from build123d import *

# Parameters (mm, degrees)
F1_DEPTH = 63.5
F2_DEPTH = 25.4
F3_DEPTH = 7.9375
F4_DEPTH = 25.4


with BuildPart() as f1:
    # F0 (on Front) → F1 (new body, symmetric)
    with BuildSketch(Plane.XZ):
        Polygon((-41.275, 9.525), (-41.275, -9.525), (41.275, -9.525), (41.275, 9.525), (22.225, 9.525), align=None)
    extrude(amount=F1_DEPTH, both=True)

    # F0 (on Front) → F2 (join, symmetric)
    with BuildSketch(Plane.XZ):
        with BuildLine():
            Line((22.225, 9.525), (41.275, 9.525))
            Line((41.275, 9.525), (41.275, 33.834597))
            ThreePointArc((41.275, 33.834597), (43.881091, 40.126257), (50.172751, 42.732348))
            Line((50.172751, 42.732348), (63.788638, 42.732348))
            Line((63.788638, 42.732348), (63.788638, 61.565076))
            Line((63.788638, 61.565076), (77.687105, 61.565076))
            Line((77.687105, 61.565076), (77.685953, 61.782348))
            Line((77.685953, 61.782348), (50.172751, 61.782348))
            ThreePointArc((50.172751, 61.782348), (30.410707, 53.596641), (22.225, 33.834597))
            Line((22.225, 33.834597), (22.225, 9.525))
        make_face()
    extrude(amount=F2_DEPTH, both=True)

    # F0 (on Front) → F3 (join, symmetric)
    with BuildSketch(Plane.XZ):
        with BuildLine():
            add(Edge.make_bspline(
                [(-41.275, 9.525), (-36.848798, 45.56419), (7.302681, 62.255602), (50.172751, 61.782348)],
                knots=[0, 0, 0, 0, 105.325787, 105.325787, 105.325787, 105.325787], degree=3))
            Line((-41.275, 9.525), (22.225, 9.525))
            Line((22.225, 9.525), (22.225, 33.834597))
            ThreePointArc((22.225, 33.834597), (30.410707, 53.596641), (50.172751, 61.782348))
        make_face()
    extrude(amount=F3_DEPTH, both=True)

    # F0 (on Front) → F4 (join, symmetric)
    with BuildSketch(Plane.XZ):
        Polygon((114.588638, 61.565076), (77.687105, 61.565076), (77.837355, 33.214565), (114.588638, 33.214565), align=None)
        Polygon((77.837355, 33.214565), (77.687105, 61.565076), (63.788638, 61.565076), (63.788638, 42.732348), (63.788638, 33.214565), align=None)
    extrude(amount=F4_DEPTH, both=True)


solid = f1.part
Design review of the part built by this model. Coordinates are the model's own, in mm. A direction names the side the tool comes from. Coordinates: 2 decimals unless noted, no trailing zeros. Order: outer loops, then holes, each group sorted by start corner. A loop starts at its lowest first (then second) coordinate and runs counter-clockwise, first axis right, second up.
Item 1: The part is to be moulded in two halves that separate along X. For faces 6 (the flat face through (114.589, 0, 47)), 7 (the cylindrical face through (30.629, 16.547, 53.813)), 8 (the flat face through (89, 0, 33.215)), 9 (the flat face through (57, 0, 42.732)), say which applies: pulls with the +X half, pulls with the -X half, needs draft (parallel to the pull), parting line crosses it, or undercut.
Item 2: For faces 1 (the flat face through (63.789, 0, 38)), 2 (the flat face through (96, 0, 61.565)), 3 (the flat face through (-5, -7.938, 30)), 4 (the flat face through (-5, 7.938, 30)), 5 (the flat face through (68, -25.4, 42)), list the 3-axis set-ups (+Z, -Z, +X, -X, +Y, -Y) from which the entire face can be reached by the end or side of a thin tool; tool diameter is ignored.
Item 3: Take a section at B-B, the plane x = 59. Write out the cut boundary in (y, z).
Item 4: For pin 1 Ø12 at (x, y) = (62.5, -17) entering from -Z; pin 2 Ø10 at (x, z) = (70.5, 31.5) entering from +Y; pin 3 Ø6 at (x, z) = (11, 17) entering from +Y, all flat-tipped, find the tip position at first contact; note any pin that passes through.
Item 5: For line 1 (X direction, y = 17.5, z = 33.5) (3 decimals); line 2 (X direction, y = 20, z = 22.5) (3 decimals); line 3 (Y direction, x = 65.5, z = 49.5), list the stretches that pass through material, from the lowest coordinate up.
Item 6: Take a section at A-A, the plane z = 1. Write out the cut boundary in (x, y) (3 decimals), then the cut area to 3 significant figures.
The answers:
1. face 6: pulls with the +X half
1. face 7: pulls with the -X half
1. face 8: needs draft
1. face 9: undercut
2. face 1: -Z, +Y, -Y
2. face 2: +Z, +X, +Y, -Y
2. face 3: +Z, -X, -Y
2. face 4: +Z, -X, +Y
2. face 5: +Z, +X, -X, -Y
3. outline: (-25.4, 42.73) - (25.4, 42.73) - (25.4, 61.78) - (-25.4, 61.78) - close
4. pin 1: stops at z = 33.21
4. pin 2: stops at y = 25.4
4. pin 3: stops at y = 7.94
5. line 1: x = 22.225 to 41.275, 63.789 to 114.589
5. line 2: x = 22.225 to 41.275
5. line 3: y = -25.4 to 25.4
6. outline: (-41.275, -63.5) - (41.275, -63.5) - (41.275, 63.5) - (-41.275, 63.5) - close
6. area: 10,500 mm2
